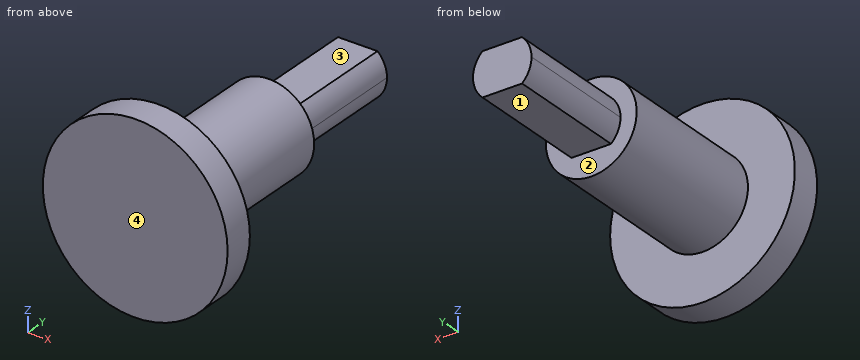
```python
from build123d import *

# Parameters (mm, degrees)
F1_DEPTH = 10.16
F2_R     = 3.7465
F3_DEPTH = 12.7
F4_R     = 7.62
F5_DEPTH = 2.54


with BuildPart() as f1:
    # F0 (on Front) → F1 (new body)
    with BuildSketch(Plane.XZ):
        with BuildLine():
            Line((-2.413, 0), (0, 0))
            Line((0, 0), (0, 1.778))
            Line((0, 1.778), (-1.631345, 1.778))
            ThreePointArc((-1.631345, 1.778), (-2.208959, 0.971117), (-2.413, 0))
        make_face()
        with BuildLine():
            Line((2.413, 0), (0, 0))
            Line((0, 0), (0, -1.778))
            Line((0, -1.778), (1.631345, -1.778))
            ThreePointArc((1.631345, -1.778), (2.208959, -0.971117), (2.413, 0))
        make_face()
        with BuildLine():
            Line((0, -1.778), (0, 0))
            Line((0, 0), (-2.413, 0))
            ThreePointArc((-2.413, 0), (-2.208959, -0.971117), (-1.631345, -1.778))
            Line((-1.631345, -1.778), (0, -1.778))
        make_face()
        with BuildLine():
            Line((0, 1.778), (0, 0))
            Line((0, 0), (2.413, 0))
            ThreePointArc((2.413, 0), (2.208959, 0.971117), (1.631345, 1.778))
            Line((1.631345, 1.778), (0, 1.778))
        make_face()
    extrude(amount=F1_DEPTH)

    # F2 (on face) → F3 (join)
    with BuildSketch(Plane.XZ.offset(10.16)):
        Circle(F2_R)
    extrude(amount=F3_DEPTH)

    # F4 (on face) → F5 (join)
    with BuildSketch(Plane.XZ.offset(22.86)):
        Circle(F4_R)
    extrude(amount=F5_DEPTH)


solid = f1.part
```
For this review, take the finished solid that the model builds, in its own axes (mm). Face numbers are marked on the shaded views. A direction names the side the tool comes from. Round coordinates to 2 decimals unless told otherwise and drop trailing zeros. Order: outer loops, then holes, each group sorted by start corner. A loop starts at its lowest first (then second) coordinate and runs counter-clockwise, first axis right, second up.
Q1. We need section B-B, the plane y = -7.5. Give the boundary of the cut face in (x, z).
Findings below:
outline: (-2.41, 0) arc R2.41 ccw to (-1.63, -1.78) - (1.63, -1.78) arc R2.41 ccw to (2.41, 0) arc R2.41 ccw to (1.63, 1.78) - (-1.63, 1.78) arc R2.41 ccw to start
Q2. Insertion check: P1, Ø6, axis at x = 0.5, y = -8, coming from the +Z side; P2, Ø2, axis at y = -22.5, z = -1.5, coming from the +X side; P3, Ø3, axis at y = -5, z = 2, coming from the -X side. Each pin has a flat end and moves straight along its axis. Give the tip position at first contact, or say it passes through.
Findings below:
P1: stops at z = 3.75
P2: stops at x = 7.6
P3: stops at x = -2.36
Q3. Wall thickness on line 1 (Y direction, x = -1.5, z = -4); line 2 (Y direction, x = 0.5, z = 2.75); line 3 (Z direction, x = -3, y = -12.75): over which ranges is each line inside the solid? List them lowest first.
Findings below:
line 1: y = -25.4 to -22.86
line 2: y = -25.4 to -10.16
line 3: z = -2.24 to 2.24
Q4. Machinability: for the marked faces 1, 2, 3 and 4, which of the approach directions +Z, -Z, +X, -X, +Y, -Y give a long, thin tool a straight path to every point of the face, cutting with its end or side? Answer none if there is none.
Findings below:
face 1: -Z, +X, -X, +Y
face 2: +Y
face 3: +Z, +X, -X, +Y
face 4: +Z, -Z, +X, -X, -Y
Q5. We need section C-C, the plane z = 0.75. Give the boundary of the cut face in (x, y).
Findings below:
outline: (-7.58, -25.4) - (7.58, -25.4) - (7.58, -22.86) - (3.67, -22.86) - (3.67, -10.16) - (2.29, -10.16) - (2.29, 0) - (-2.29, 0) - (-2.29, -10.16) - (-3.67, -10.16) - (-3.67, -22.86) - (-7.58, -22.86) - close
Q6. We need section A-A, the plane x = 0. Give the boundary of the cut face in (y, z).
Findings below:
outline: (-25.4, -7.62) - (-22.86, -7.62) - (-22.86, -3.75) - (-10.16, -3.75) - (-10.16, -1.78) - (0, -1.78) - (0, 1.78) - (-10.16, 1.78) - (-10.16, 3.75) - (-22.86, 3.75) - (-22.86, 7.62) - (-25.4, 7.62) - close
Q7. We need section D-D, the plane y = -19. Give the boundary of the cut face in (x, z), plus the area to 3 significant figures.
Findings below:
outline: circle Ø7.49 at (0, 0)
area: 44.1 mm2
